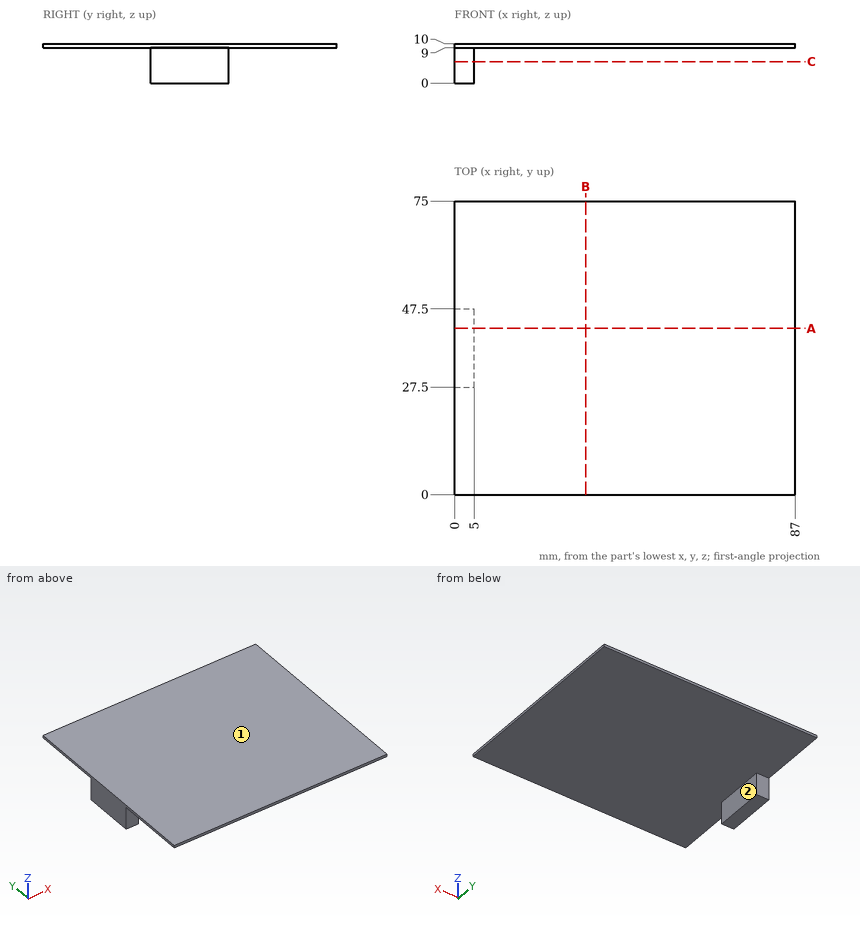
Check sheet for the drawn part. Datum: minimum x, y, z corner. Units: mm. A direction names the side the tool comes from. Coordinates: 2 decimals unless noted, no trailing zeros. Loops run counter-clockwise (first coordinate to the right, second up) from the corner with the lowest first, then second, coordinate; pieces in that order, holes last. Notation, with made-up numbers: (-32.75, 71.25) -> (19.25, 71.25) arc R18 cw to (19.25, 80.25) -> close; hole circle Ø9 at (30, -35). An arc over 180 degrees is marked (long way). Answer in a Markdown table with one row per item.
1) Section check C-C (z = 5.5). Record the cut outline in (x, y), and give its area (3 significant figures).
The answers:
| item | result |
|---|---|
| outline | (0, 27.5) -> (5, 27.5) -> (5, 47.5) -> (0, 47.5) -> close |
| area | 100 mm2 |
2) Access from +Z, -Z, +X, -X, +Y, -Y to the whole of each face (thin tool, end or side, straight path). Record for the marked faces 1 and 2.
The answers:
| item | result |
|---|---|
| face 1 | +Z, +X, -X, +Y, -Y |
| face 2 | -Z, +X, +Y, -Y |
3) Section check A-A (y = 42.5). Record the cut outline in (x, z).
The answers:
| item | result |
|---|---|
| outline | (0, 0) -> (5, 0) -> (5, 9) -> (87, 9) -> (87, 10) -> (0, 10) -> close |
4) Scan lines: line 1 along X through (y, z) = (34, 5.25); line 2 along Z through (x, y) = (50, 8.5). Record each from-to range of solid material in increasing order. Write a range as from..to.
The answers:
| item | result |
|---|---|
| line 1 | x = 0..5 |
| line 2 | z = 9..10 |
5) Section check B-B (x = 33.5). Record the cut outline in (y, z).
The answers:
| item | result |
|---|---|
| outline | (0, 9) -> (75, 9) -> (75, 10) -> (0, 10) -> close |
6) Depth check by flat-ended pin: P1, Ø1.5, axis at x = 2.5, z = 6, coming from the -Y side; P2, Ø1.5, axis at x = 2.5, z = 3.5, coming from the +Y side. Enter the tip coordinate at first touch or a pass-through.
The answers:
| item | result |
|---|---|
| P1 | stops at y = 27.5 |
| P2 | stops at y = 47.5 |
